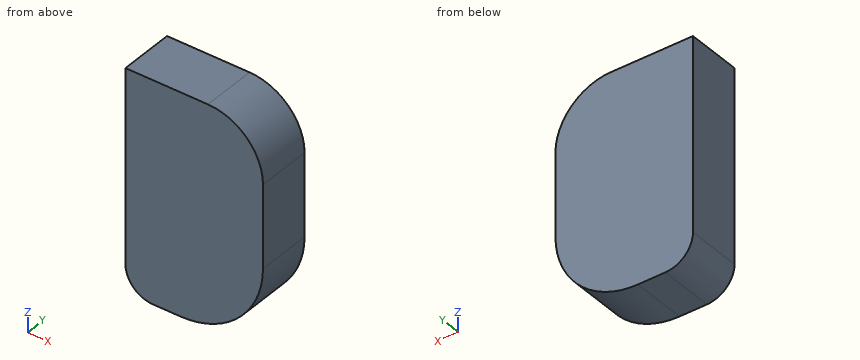
Autodesk Inventor part; units mm, degrees
ref_plane "YZ Plane" through (0, 0, 0) normal (1, 0, 0) x (0, 1, 0)
ref_plane "XZ Plane" through (0, 0, 0) normal (0, 1, 0) x (-1, 0, 0)
ref_plane "XY Plane" through (0, 0, 0) normal (0, 0, 1) x (1, 0, 0)
sketch "Sketch1" plane through (0, 0, 0) normal (0, 1, 0) x (-1, 0, 0)
  line L0 (0, 0) -> (-31.75, 0)
  line L1 (-31.75, 0) -> (-31.75, 50.8)
  line L2 (-31.75, 50.8) -> (0, 50.8)
  line L3 (0, 50.8) -> (0, 0)
  dimension "d0" = 31.75
  dimension "d1" = 50.8
extrude "Extrusion1" add sketch "Sketch1" along normal blind 12.7
fillet "Fillet1" radius 6.35 1 edges at (0, 6.35, 0)
fillet "Fillet2" radius 12.7 1 edges at (31.75, 6.35, 50.8)
fillet "Fillet3" radius 19.05 1 edges at (31.75, 6.35, 0)
properties part number "Practice1"
The model under review builds one solid part; all positions refer to its coordinate system, in mm. Coordinates: 2 decimals unless noted, no trailing zeros. Order: outer loops, then holes, each group sorted by start corner. A loop starts at its lowest first (then second) coordinate and runs counter-clockwise, first axis right, second up. Notation, with made-up numbers: (38, -22.5) -> (44, -22.5) arc R23 ccw to (44, 16.5) -> close; hole circle Ø4 at (15, 20). An arc over 180 degrees is marked (long way). Answer in a Markdown table with one row per item. Add a question column.
Item 1: To check wall thickness, follow probe 1 along Z at (x, y) = (29.5, 4.25); probe 2 along X at (y, z) = (3.25, 18.5); probe 3 along Z at (x, y) = (16, 2.75). State the ranges of each line that lie inside material, in increasing order.
Item 2: We need section C-C on z = 43.5. Write out the cut boundary in (x, y).
Item 3: We need section B-B on x = 25. Write out the cut boundary in (y, z), plus the area to 3 significant figures.
Item 4: Clearance check with flat-ended pins moving along their axes: pin 1 (3 mm diameter, centred on x = 4.5, y = 9, fed in from -Z); pin 2 (3 mm diameter, centred on x = 20.5, y = 8.5, fed in from -Z). State where each tip first meets the part, or that it passes through.
Item 5: We need section A-A on y = 9. Write out the cut boundary in (x, z).
Final values:
| question | item | result |
|---|---|---|
| 1 | probe 1 | z = 10.07 to 45.32 |
| 1 | probe 2 | x = 0 to 31.74 |
| 1 | probe 3 | z = 0.29 to 50.8 |
| 2 | outline | (0, 0) -> (30.54, 0) -> (30.54, 12.7) -> (0, 12.7) -> close |
| 3 | outline | (0, 4.5) -> (12.7, 4.5) -> (12.7, 49.32) -> (0, 49.32) -> close |
| 3 | area | 569 mm2 |
| 4 | pin 1 | stops at z = 0.01 |
| 4 | pin 2 | stops at z = 1.07 |
| 5 | outline | (0, 6.35) arc R6.35 ccw to (6.35, 0) -> (12.7, 0) arc R19.05 ccw to (31.75, 19.05) -> (31.75, 38.1) arc R12.7 ccw to (19.05, 50.8) -> (0, 50.8) -> close |
